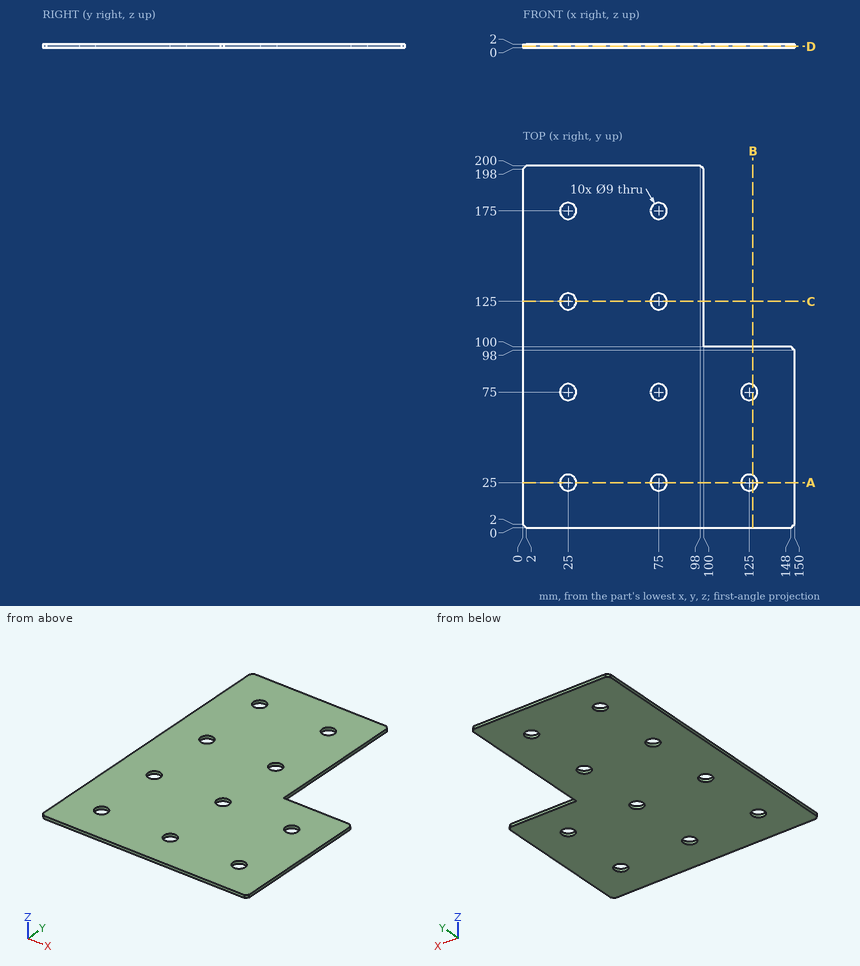
The drawing under review shows one solid part. Ordinate dimensions are in mm from its lowest x, y, z. Round coordinates to 2 decimals unless told otherwise and drop trailing zeros. Loops run counter-clockwise (first coordinate to the right, second up) from the corner with the lowest first, then second, coordinate; pieces in that order, holes last. Notation, with made-up numbers: (55, -34) - (66, -34) arc R24 ccw to (66, -18) - close; hole circle Ø7 at (86.5, 49.25). An arc over 180 degrees is marked (long way). One line per item, written item: value. Start each with the question number.
1) To check wall thickness, follow L1, parallel to Y at x = 25, z = 0.65; L2, parallel to Y at x = 125, z = 1.4; L3, parallel to Y at x = 127.5, z = 1.7. State the ranges of each line that lie inside material, in increasing order. Write a range as from..to.
2) Consider section C-C on y = 125. Give the boundary of the cut face in (x, z), then the cut area to 3 significant figures.
3) Consider section B-B on x = 127. Give the boundary of the cut face in (y, z), then the cut area to 3 significant figures.
4) Consider section A-A on y = 25. Give the boundary of the cut face in (x, z).
5) Consider section D-D on z = 0.7. Give the number of separate pieces and of enclosed holes in the cut face, then the cut area to 3 significant figures.
6) Insertion check: pin 1 Ø0.6 at (y, z) = (159.5, 1) entering from +X; pin 2 Ø0.6 at (x, z) = (120.5, 0.5) entering from +Y. Each pin has a flat end and moves straight along its axis. Give the tip position at first contact, or say it passes through.
Reported:
1. L1: y = 0..20.5, 29.5..70.5, 79.5..120.5, 129.5..170.5, 179.5..200
1. L2: y = 0..20.5, 29.5..70.5, 79.5..100
1. L3: y = 0..21.26, 28.74..71.26, 78.74..100
2. outline: (0, 0) - (20.5, 0) - (20.5, 2) - (0, 2) - close; (29.5, 0) - (70.5, 0) - (70.5, 2) - (29.5, 2) - close; (79.5, 0) - (100, 0) - (100, 2) - (79.5, 2) - close
2. area: 164 mm^2
3. outline: (0, 0) - (20.97, 0) - (20.97, 2) - (0, 2) - close; (29.03, 0) - (70.97, 0) - (70.97, 2) - (29.03, 2) - close; (79.03, 0) - (100, 0) - (100, 2) - (79.03, 2) - close
3. area: 168 mm^2
4. outline: (0, 0) - (20.5, 0) - (20.5, 2) - (0, 2) - close; (29.5, 0) - (70.5, 0) - (70.5, 2) - (29.5, 2) - close; (79.5, 0) - (120.5, 0) - (120.5, 2) - (79.5, 2) - close; (129.5, 0) - (150, 0) - (150, 2) - (129.5, 2) - close
5. separate pieces: 1
5. enclosed holes: 10
5. area: 24,400 mm^2
6. pin 1: stops at x = 100
6. pin 2: stops at y = 100
